The model under review builds one solid part; all positions refer to its coordinate system, in mm. Face numbers are marked on the shaded views. Round coordinates to 2 decimals unless told otherwise and drop trailing zeros. Order: outer loops, then holes, each group sorted by start corner. A loop starts at its lowest first (then second) coordinate and runs counter-clockwise, first axis right, second up. Notation, with made-up numbers: M 67.5,41.25 L 99.5,41.25 A34 ccw 99.5,77.25 Z; hole C 53.5,-31 d8. An arc over 180 degrees is marked long. One line per item, written item: value. Start each with the question number.
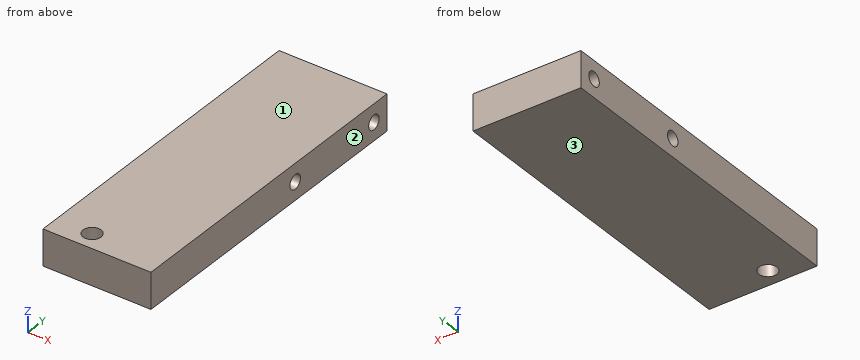
from build123d import *

# Parameters (mm, degrees)
SKETCH1_W           = 30
SKETCH1_H           = 90
BOSS_EXTRUDE1_DEPTH = 10
CUT_EXTRUDE2_REACH  = 97.394
SKETCH4_R           = 2.5
SKETCH3_R           = 2
CUT_EXTRUDE3_DEPTH  = 96.393920142


with BuildPart() as part:
    # Sketch1 → Boss-Extrude1 (new body)
    with BuildSketch(Plane.XY):
        with Locations((15, 45)):
            Rectangle(SKETCH1_W, SKETCH1_H)
    extrude(amount=BOSS_EXTRUDE1_DEPTH)

    # Sketch4 → Cut-Extrude2 (cut, up to next)
    with BuildSketch(Plane.XY.offset(10), mode=Mode.PRIVATE) as cut_extrude2_sk1:
        with Locations((10, 5)):
            Circle(SKETCH4_R)
    cut_extrude2_tool1 = extrude(cut_extrude2_sk1.sketch, amount=-CUT_EXTRUDE2_REACH, mode=Mode.PRIVATE) & part.part
    add(cut_extrude2_tool1.solids().sort_by_distance((10, 5, 10))[0], mode=Mode.SUBTRACT)

    # Sketch3 → Cut-Extrude3 (cut, through all)
    with BuildSketch(Plane(origin=(30, 0, 0), x_dir=(0, 0, -1), z_dir=(1, 0, 0))):
        with Locations((-5, 85)):
            Circle(SKETCH3_R)
        with Locations((-5, 55)):
            Circle(SKETCH3_R)
    extrude(amount=-CUT_EXTRUDE3_DEPTH, mode=Mode.SUBTRACT)


solid = part.part
Item 1: Consider section C-C, the plane y = 5. Give the boundary of the cut face in (x, z), then the cut area to 3 significant figures.
Item 2: Consider section D-D, the plane x = 5.5. Give the boundary of the cut face in (y, z), then the cut area to 3 significant figures.
Item 3: The part is to be moulded in two halves that separate along Z. For the marked faces 1, 2 and 3, say which applies: pulls with the +Z half, pulls with the -Z half, needs draft (parallel to the pull), parting line crosses it, or undercut.
Item 4: Consider section B-B, the plane z = 4.5. Give the boundary of the cut face in (x, y).
Item 5: Wall thickness on L1, parallel to Y at x = 21, z = 5; L2, parallel to Y at x = 27, z = 4.5; L3, parallel to Y at x = 9.25, z = 5.5: over which ranges is each line inside the solid? List them lowest first.
Item 6: Consider section A-A, the plane x = 10. Give the boundary of the cut face in (y, z).
Computed:
1. outline: M 0,0 L 7.5,0 L 7.5,10 L 0,10 Z; M 12.5,0 L 30,0 L 30,10 L 12.5,10 Z
1. area: 250 mm^2
2. outline: M 0,0 L 90,0 L 90,10 L 0,10 Z; hole C 55,5 d4; hole C 85,5 d4
2. area: 875 mm^2
3. face 1: pulls with the +Z half
3. face 2: needs draft
3. face 3: pulls with the -Z half
4. outline: M 0,0 L 30,0 L 30,53.06 L 0,53.06 Z; M 0,56.94 L 30,56.94 L 30,83.06 L 0,83.06 Z; M 0,86.94 L 30,86.94 L 30,90 L 0,90 Z; hole C 10,5 d5
5. L1: y = 0 to 53, 57 to 83, 87 to 90
5. L2: y = 0 to 53.06, 56.94 to 83.06, 86.94 to 90
5. L3: y = 0 to 2.62, 7.38 to 53.06, 56.94 to 83.06, 86.94 to 90
6. outline: M 0,0 L 2.5,0 L 2.5,10 L 0,10 Z; M 7.5,0 L 90,0 L 90,10 L 7.5,10 Z; hole C 55,5 d4; hole C 85,5 d4
